Design review of the part shown in the three views and the two pictorial views. Dimensions are in mm from the part's minimum x, y and z. Give positions to 0.01 mm unless a question says otherwise; leave off trailing zeros. Order: outer loops, then holes, each group sorted by start corner. A loop starts at its lowest first (then second) coordinate and runs counter-clockwise, first axis right, second up. Notation, with made-up numbers: M -33,-38.75 L -23,-38.75 A27 ccw -23,-10.75 Z; hole C 55,51 d10. An arc over 180 degrees is marked long. Answer as a JSON object with one key per item and string values.
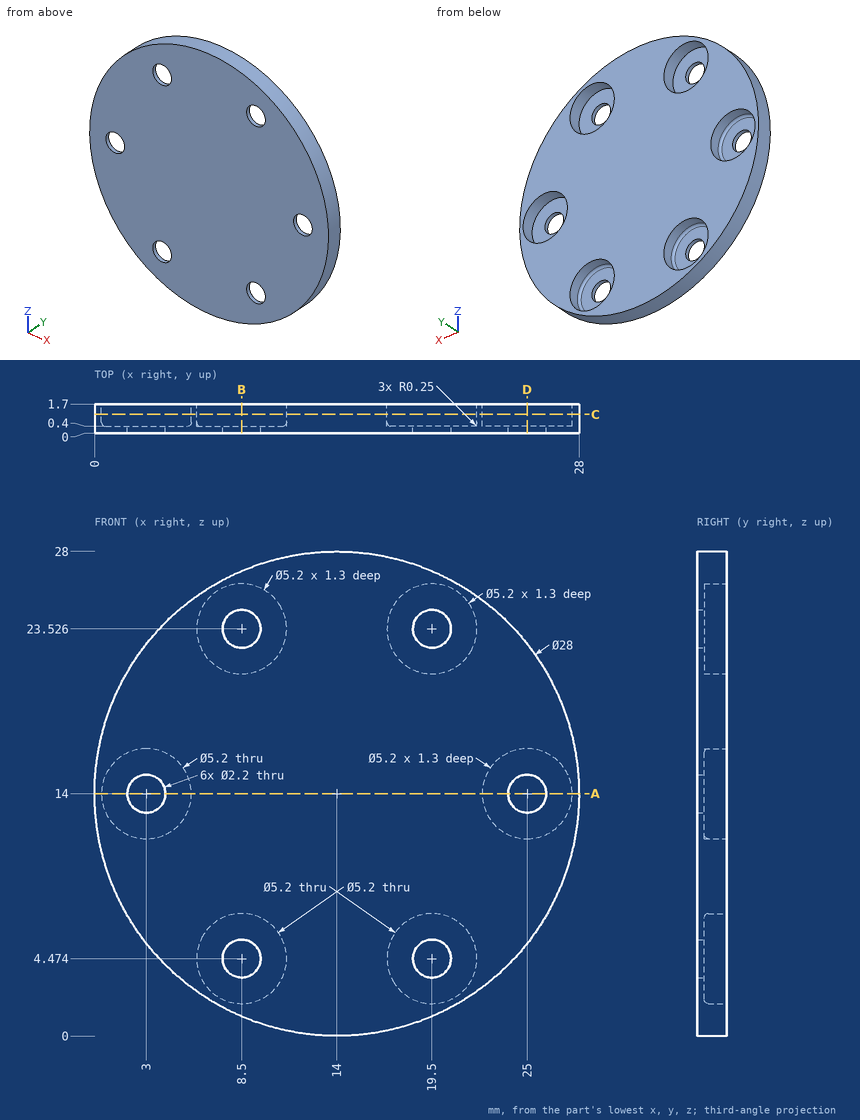
(1) We need section C-C (y = 1.1). Write out the cut boundary in (x, z), plus the area to 3 significant figures.
Checked values:
{"outline": "C 14,14 d28; hole C 3,14 d5.2; hole C 8.5,4.47 d5.2; hole C 8.5,23.53 d5.2; hole C 19.5,4.47 d5.2; hole C 19.5,23.53 d5.2; hole C 25,14 d5.2", "area": "488 mm^2"}
(2) We need section D-D (x = 25). Write out the cut boundary in (y, z).
Checked values:
{"outline": "M 0,5.34 L 1.7,5.34 L 1.7,11.4 L 0.4,11.4 L 0.4,12.9 L 0,12.9 Z; M 0,15.1 L 0.4,15.1 L 0.4,16.6 L 1.7,16.6 L 1.7,22.66 L 0,22.66 Z"}
(3) To check wall thickness, follow L1, parallel to X at y = 0.2, z = 14; L2, parallel to X at y = 1.1, z = 24.25 (1 decimal); L3, parallel to Y at x = 19, z = 6.5. State the ranges of each line that lie inside material, in increasing order. Write a range as from..to.
Checked values:
{"L1": "x = 0..1.9, 4.1..23.9, 26.1..28", "L2": "x = 4.5..6, 11..17, 22..23.5", "L3": "y = 0..0.4"}
(4) Insertion check: pin 1 (3.5 mm diameter, centred on x = 3, z = 14, fed in from +Y); pin 2 (1.8 mm diameter, centred on x = 25, z = 14, fed in from -Y); pin 3 (1 mm diameter, centred on x = 7, y = 1.5, fed in from -Z). Each pin has a flat end and moves straight along its axis. Give the tip position at first contact, or say it passes through.
Checked values:
{"pin 1": "stops at y = 0.4", "pin 2": "passes through", "pin 3": "stops at z = 1.6"}
(5) We need section A-A (z = 14). Write out the cut boundary in (x, y).
Checked values:
{"outline": "M 0,0 L 1.9,0 L 1.9,0.4 L 0.65,0.4 A0.25 cw 0.4,0.65 L 0.4,1.7 L 0,1.7 Z; M 4.1,0 L 23.9,0 L 23.9,0.4 L 22.4,0.4 L 22.4,1.7 L 5.6,1.7 L 5.6,0.65 A0.25 cw 5.35,0.4 L 4.1,0.4 Z; M 26.1,0 L 28,0 L 28,1.7 L 27.6,1.7 L 27.6,0.4 L 26.1,0.4 Z"}
(6) We need section B-B (x = 8.5). Write out the cut boundary in (y, z).
Checked values:
{"outline": "M 0,1.13 L 1.7,1.13 L 1.7,1.87 L 0.65,1.87 A0.25 cw 0.4,2.12 L 0.4,3.37 L 0,3.37 Z; M 0,5.57 L 0.4,5.57 L 0.4,6.82 A0.25 cw 0.65,7.07 L 1.7,7.07 L 1.7,20.93 L 0.4,20.93 L 0.4,22.43 L 0,22.43 Z; M 0,24.63 L 0.4,24.63 L 0.4,26.13 L 1.7,26.13 L 1.7,26.87 L 0,26.87 Z"}
